Here's the drawing with two shaded views (mm, measured from the low corner). I have some questions. A direction names the side the tool comes from. Round coordinates to 2 decimals unless told otherwise and drop trailing zeros. Loops run counter-clockwise (first coordinate to the right, second up) from the corner with the lowest first, then second, coordinate; pieces in that order, holes last.
(1) I want a section at D-D on z = 20. Write out the boundary of the cut face in (x, y), plus the area to 3 significant figures.
(2) Will these pins go through, and if not, where does the flat tip stop? pin 1 Ø4 at (x, y) = (30, 6) entering from -Z; pin 2 Ø6 at (y, z) = (8, 11) entering from -X; pin 3 Ø6 at (y, z) = (3, 21.5) entering from +X; pin 4 Ø3 at (x, y) = (2, 6) entering from +Z.
(3) I want a section at B-B on y = 6. Write out the boundary of the cut face in (x, z), plus the area to 3 significant figures.
(4) If I drill on line 1 along Y through (x, z) = (2, 16.6); line 2 along Y through (x, z) = (9.5, 15.5); line 3 along Z through (x, y) = (18.5, 6.25), over which ranges is the centre line in solid material (lowest first)?
(5) Which directions (+Z, -Z, +X, -X, +Y, -Y) give clear straight access to the entire face, cutting with the end or side of a thin tool? Please do the marked faces 1, 2, 3 and 4.
(6) I want a section at C-C on y = 10.75. Write out the boundary of the cut face in (x, z), plus the area to 3 significant figures.
(7) I want a section at A-A on x = 9.5. Write out the boundary of the cut face in (y, z).
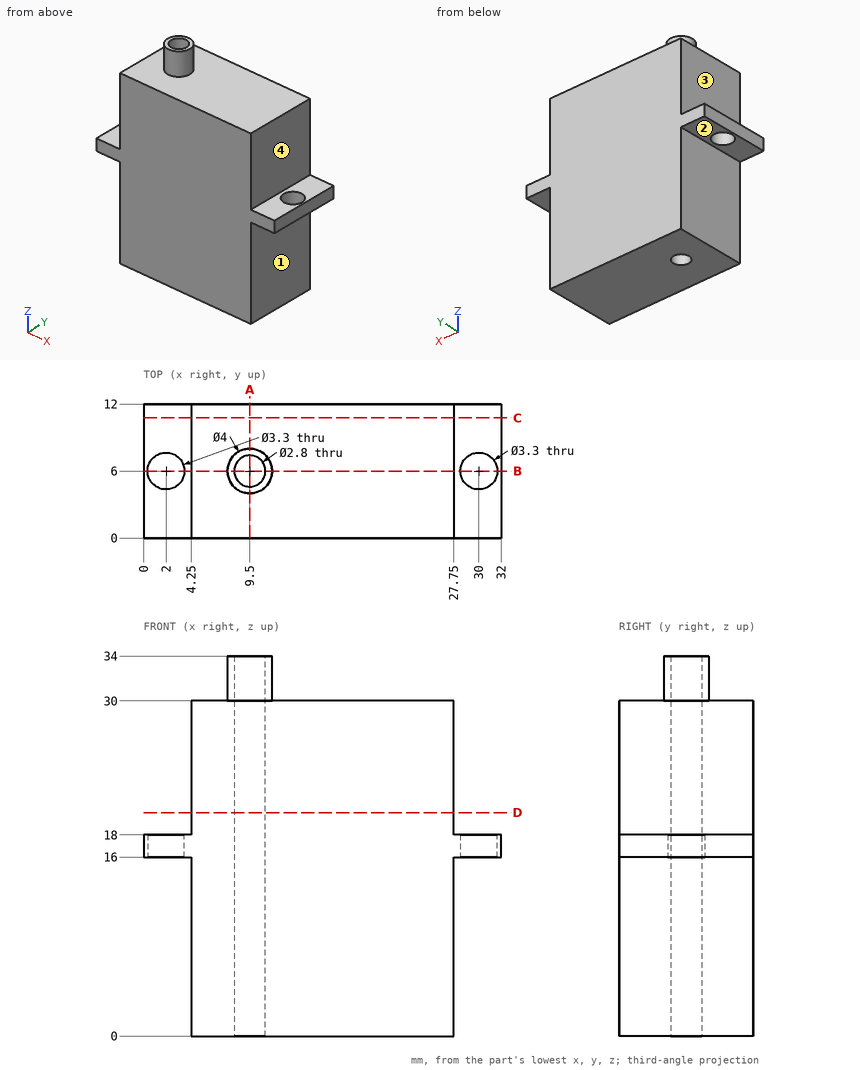
Filled sheet:
1. outline: (4.25, 0) - (27.75, 0) - (27.75, 12) - (4.25, 12) - close; hole circle Ø2.8 at (9.5, 6)
1. area: 276 mm2
2. pin 1: stops at z = 16
2. pin 2: stops at x = 4.25
2. pin 3: stops at x = 27.75
2. pin 4: passes through
3. outline: (0, 16) - (0.35, 16) - (0.35, 18) - (0, 18) - close; (3.65, 16) - (4.25, 16) - (4.25, 0) - (8.1, 0) - (8.1, 34) - (7.5, 34) - (7.5, 30) - (4.25, 30) - (4.25, 18) - (3.65, 18) - close; (10.9, 0) - (27.75, 0) - (27.75, 16) - (28.35, 16) - (28.35, 18) - (27.75, 18) - (27.75, 30) - (11.5, 30) - (11.5, 34) - (10.9, 34) - close; (31.65, 16) - (32, 16) - (32, 18) - (31.65, 18) - close
3. area: 630 mm2
4. line 1: y = 0 to 4.35, 7.65 to 12
4. line 2: y = 0 to 4.6, 7.4 to 12
4. line 3: z = 0 to 30
5. face 1: -Z, +X, +Y, -Y
5. face 2: -Z, -X, +Y, -Y
5. face 3: +Z, -X, +Y, -Y
5. face 4: +Z, +X, +Y, -Y
6. outline: (0, 16) - (4.25, 16) - (4.25, 0) - (27.75, 0) - (27.75, 16) - (32, 16) - (32, 18) - (27.75, 18) - (27.75, 30) - (4.25, 30) - (4.25, 18) - (0, 18) - close
6. area: 722 mm2
7. outline: (0, 0) - (4.6, 0) - (4.6, 34) - (4, 34) - (4, 30) - (0, 30) - close; (7.4, 0) - (12, 0) - (12, 30) - (8, 30) - (8, 34) - (7.4, 34) - close
